from build123d import *

# Parameters (mm, degrees)
F1_DEPTH  = 714.375
F3_D      = 22.225
F3_DEPTH  = 76.2
F3_TIP    = 6.6770636289
F5_DEPTH  = 1792.224
F6_W      = 304.8
F6_H      = 307.975
F7_DEPTH  = 19.05
F10_D     = 22.225
F10_DEPTH = 76.2
F10_TIP   = 6.6770636289
F11_W     = 19.05
F11_H     = 277.495
F12_DEPTH = 304.8
F13_W     = 19.05
F13_H     = 277.495
F14_DEPTH = 304.8
F16_D     = 41.402
F18_DEPTH = 168.402
F19_W     = 304.8
F19_H     = 307.848
F20_DEPTH = 19.05
F22_D     = 28.448
F22_2_D   = 28.448
F24_W     = 19.05
F24_H     = 457.2
F25_DEPTH = 168.402
F27_DEPTH = 1260.349


# Not quite as in the source:
# - a length typed as a fraction of an inch, garbled in the dataset ("3 / 203.2 mm" for 3/8 in), is restored


with BuildPart() as f1:
    # F0 (on Right) → F1 (new body, symmetric)
    with BuildSketch(Plane.YZ):
        with BuildLine():
            Line((152.4, 153.9875), (-152.4, 153.9875))
            Line((-152.4, 153.9875), (-152.4, 138.7475))
            Line((-152.4, 138.7475), (-19.05, 138.7475))
            ThreePointArc((-19.05, 138.7475), (-10.0697438789, 135.0277561211), (-6.35, 126.0475))
            Line((-6.35, 126.0475), (-6.35, -126.0475))
            ThreePointArc((-6.35, -126.0475), (-10.0697438789, -135.0277561211), (-19.05, -138.7475))
            Line((-19.05, -138.7475), (-152.4, -138.7475))
            Line((-152.4, -138.7475), (-152.4, -153.9875))
            Line((-152.4, -153.9875), (152.4, -153.9875))
            Line((152.4, -153.9875), (152.4, -138.7475))
            Line((152.4, -138.7475), (19.05, -138.7475))
            ThreePointArc((19.05, -138.7475), (10.0697438789, -135.0277561211), (6.35, -126.0475))
            Line((6.35, -126.0475), (6.35, 126.0475))
            ThreePointArc((6.35, 126.0475), (10.0697438789, 135.0277561211), (19.05, 138.7475))
            Line((19.05, 138.7475), (152.4, 138.7475))
            Line((152.4, 138.7475), (152.4, 153.9875))
        make_face()
    extrude(amount=F1_DEPTH, both=True)

    # F3
    with Locations(Plane.XY.offset(153.9875)):
        with Locations((-381, 82.55), (-381, -82.55), (171.45, 82.55), (171.45, -82.55), (615.95, 82.55), (615.95, -82.55)):
            Hole(F3_D / 2, depth=F3_DEPTH)
            with Locations((0, 0, -(F3_DEPTH + F3_TIP / 2))):  # 118° drill point
                Cone(0, F3_D / 2, F3_TIP, mode=Mode.SUBTRACT)


with BuildPart() as f5:
    # F4 (on Front) → F5 (new body)
    with BuildSketch(Plane.XZ):
        with BuildLine():
            Line((-47.625, 153.9875), (-352.425, 153.9875))
            Line((-352.425, 153.9875), (-352.425, 138.7475))
            Line((-352.425, 138.7475), (-219.075, 138.7475))
            ThreePointArc((-219.075, 138.7475), (-210.0947438789, 135.0277561211), (-206.375, 126.0475))
            Line((-206.375, 126.0475), (-206.375, -126.0475))
            ThreePointArc((-206.375, -126.0475), (-210.0947438789, -135.0277561211), (-219.075, -138.7475))
            Line((-219.075, -138.7475), (-352.425, -138.7475))
            Line((-352.425, -138.7475), (-352.425, -153.9875))
            Line((-352.425, -153.9875), (-47.625, -153.9875))
            Line((-47.625, -153.9875), (-47.625, -138.7475))
            Line((-47.625, -138.7475), (-180.975, -138.7475))
            ThreePointArc((-180.975, -138.7475), (-189.9552561211, -135.0277561211), (-193.675, -126.0475))
            Line((-193.675, -126.0475), (-193.675, 126.0475))
            ThreePointArc((-193.675, 126.0475), (-189.9552561211, 135.0277561211), (-180.975, 138.7475))
            Line((-180.975, 138.7475), (-47.625, 138.7475))
            Line((-47.625, 138.7475), (-47.625, 153.9875))
        make_face()
    extrude(amount=F5_DEPTH)


with BuildPart() as f5b:
    # F4 (on Front) → F5, piece 2 (new body)
    with BuildSketch(Plane.XZ):
        with BuildLine():
            Line((688.975, 153.9875), (384.175, 153.9875))
            Line((384.175, 153.9875), (384.175, 138.7475))
            Line((384.175, 138.7475), (517.525, 138.7475))
            ThreePointArc((517.525, 138.7475), (526.5052561211, 135.0277561211), (530.225, 126.0475))
            Line((530.225, 126.0475), (530.225, -126.0475))
            ThreePointArc((530.225, -126.0475), (526.5052561211, -135.0277561211), (517.525, -138.7475))
            Line((517.525, -138.7475), (384.175, -138.7475))
            Line((384.175, -138.7475), (384.175, -153.9875))
            Line((384.175, -153.9875), (688.975, -153.9875))
            Line((688.975, -153.9875), (688.975, -138.7475))
            Line((688.975, -138.7475), (555.625, -138.7475))
            ThreePointArc((555.625, -138.7475), (546.6447438789, -135.0277561211), (542.925, -126.0475))
            Line((542.925, -126.0475), (542.925, 126.0475))
            ThreePointArc((542.925, 126.0475), (546.6447438789, 135.0277561211), (555.625, 138.7475))
            Line((555.625, 138.7475), (688.975, 138.7475))
            Line((688.975, 138.7475), (688.975, 153.9875))
        make_face()
    extrude(amount=F5_DEPTH)


with BuildPart() as f7:
    # F6 (on face) → F7 (new body)
    with BuildSketch(Plane.XZ.offset(1792.224)):
        with Locations((-200.025, 0)):
            Rectangle(F6_W, F6_H)
    extrude(amount=F7_DEPTH)


with BuildPart() as f7b:
    # F6 (on face) → F7, piece 2 (new body)
    with BuildSketch(Plane.XZ.offset(1792.224)):
        with Locations((536.575, 0)):
            Rectangle(F6_W, F6_H)
    extrude(amount=F7_DEPTH)


with BuildPart() as f1_1:
    add(f1.part)

    # F8: union F5, F5b, F7b, F7
    add(f5.part)
    add(f5b.part)
    add(f7b.part)
    add(f7.part)

    # F10
    with Locations(Plane.XY.offset(153.9875)):
        with Locations((615.95, -82.55)):
            Hole(F10_D / 2, depth=F10_DEPTH)
            with Locations((0, 0, -(F10_DEPTH + F10_TIP / 2))):  # 118° drill point
                Cone(0, F10_D / 2, F10_TIP, mode=Mode.SUBTRACT)

    # F11 (on face) → F12 (join)
    with BuildSketch(Plane.YZ.offset(688.975)):
        with Locations((-1636.649, 0)):
            Rectangle(F11_W, F11_H)
    extrude(amount=-F12_DEPTH)

    # F13 (on face) → F14 (join)
    with BuildSketch(Plane(origin=(-352.425, 0, 0), x_dir=(0, -1, 0), z_dir=(-1, 0, 0))):
        with Locations((1636.649, 0)):
            Rectangle(F13_W, F13_H)
    extrude(amount=-F14_DEPTH)

    # F16 (through all)
    with Locations(Plane.XY.offset(153.9875)):
        with Locations((619.125, -1739.9), (454.025, -1739.9), (-117.475, -1739.9), (-282.575, -1739.9)):
            Hole(F16_D / 2)


with BuildPart() as f18:
    # F17 (on face) → F18 (new body)
    with BuildSketch(Plane(origin=(0, 0, -153.9875), x_dir=(1, 0, 0), z_dir=(0, 0, -1))):
        with BuildLine():
            Line((-352.425, 420.116), (-352.425, 404.876))
            Line((-352.425, 404.876), (-47.625, 404.876))
            Line((-47.625, 404.876), (-47.625, 420.116))
            Line((-47.625, 420.116), (-180.975, 420.116))
            ThreePointArc((-180.975, 420.116), (-189.9552561211, 423.8357438789), (-193.675, 432.816))
            Line((-193.675, 432.816), (-193.675, 684.784))
            ThreePointArc((-193.675, 684.784), (-189.9552561211, 693.7642561211), (-180.975, 697.484))
            Line((-180.975, 697.484), (-47.625, 697.484))
            Line((-47.625, 697.484), (-47.625, 712.724))
            Line((-47.625, 712.724), (-352.425, 712.724))
            Line((-352.425, 712.724), (-352.425, 697.484))
            Line((-352.425, 697.484), (-219.075, 697.484))
            ThreePointArc((-219.075, 697.484), (-210.0947438789, 693.7642561211), (-206.375, 684.784))
            Line((-206.375, 684.784), (-206.375, 432.816))
            ThreePointArc((-206.375, 432.816), (-210.0947438789, 423.8357438789), (-219.075, 420.116))
            Line((-219.075, 420.116), (-352.425, 420.116))
        make_face()
    extrude(amount=F18_DEPTH)


with BuildPart() as f18b:
    # F17 (on face) → F18, piece 2 (new body)
    with BuildSketch(Plane(origin=(0, 0, -153.9875), x_dir=(1, 0, 0), z_dir=(0, 0, -1))):
        with BuildLine():
            Line((688.975, 420.116), (555.625, 420.116))
            ThreePointArc((555.625, 420.116), (546.6447438789, 423.8357438789), (542.925, 432.816))
            Line((542.925, 432.816), (542.925, 684.784))
            ThreePointArc((542.925, 684.784), (546.6447438789, 693.7642561211), (555.625, 697.484))
            Line((555.625, 697.484), (688.975, 697.484))
            Line((688.975, 697.484), (688.975, 712.724))
            Line((688.975, 712.724), (384.175, 712.724))
            Line((384.175, 712.724), (384.175, 697.484))
            Line((384.175, 697.484), (517.525, 697.484))
            ThreePointArc((517.525, 697.484), (526.5052561211, 693.7642561211), (530.225, 684.784))
            Line((530.225, 684.784), (530.225, 432.816))
            ThreePointArc((530.225, 432.816), (526.5052561211, 423.8357438789), (517.525, 420.116))
            Line((517.525, 420.116), (384.175, 420.116))
            Line((384.175, 420.116), (384.175, 404.876))
            Line((384.175, 404.876), (688.975, 404.876))
            Line((688.975, 404.876), (688.975, 420.116))
        make_face()
    extrude(amount=F18_DEPTH)


with BuildPart() as f20:
    # F19 (on face) → F20 (new body)
    with BuildSketch(Plane(origin=(0, 0, -322.3895), x_dir=(1, 0, 0), z_dir=(0, 0, -1))):
        with Locations((-200.025, 558.8)):
            Rectangle(F19_W, F19_H)
    extrude(amount=F20_DEPTH)

    # F22 (through all)
    with Locations(Plane(origin=(0, 0, -341.4395), x_dir=(1, 0, 0), z_dir=(0, 0, -1))):
        with Locations((-269.1834158416, 628.65), (-130.8665841584, 628.65), (-269.1834158416, 488.95), (-130.8665841584, 488.95), (467.4165841584, 628.65), (605.7334158416, 628.65), (605.7334158416, 488.95), (467.4165841584, 488.95)):
            Hole(F22_D / 2)


with BuildPart() as f20b:
    # F19 (on face) → F20, piece 2 (new body)
    with BuildSketch(Plane(origin=(0, 0, -322.3895), x_dir=(1, 0, 0), z_dir=(0, 0, -1))):
        with Locations((536.575, 558.8)):
            Rectangle(F19_W, F19_H)
    extrude(amount=F20_DEPTH)

    # F22#2 (through all)
    with Locations(Plane(origin=(0, 0, -341.4395), x_dir=(1, 0, 0), z_dir=(0, 0, -1))):
        with Locations((-269.1834158416, 628.65), (-130.8665841584, 628.65), (-269.1834158416, 488.95), (-130.8665841584, 488.95), (467.4165841584, 628.65), (605.7334158416, 628.65), (605.7334158416, 488.95), (467.4165841584, 488.95)):
            Hole(F22_2_D / 2)


with BuildPart() as f1_2:
    add(f1_1.part)

    # F23: union F18, F20, F18b, F20b
    add(f18.part)
    add(f20.part)
    add(f18b.part)
    add(f20b.part)

    # F24 (on face) → F25 (join)
    with BuildSketch(Plane(origin=(0, 0, -153.9875), x_dir=(1, 0, 0), z_dir=(0, 0, -1))):
        with Locations((-200.152, 176.276)):
            Rectangle(F24_W, F24_H)
        with Locations((536.448, 176.276)):
            Rectangle(F24_W, F24_H)
    extrude(amount=F25_DEPTH)

    # F26 (on face) → F27 (cut, through all)
    with BuildSketch(Plane.YZ.offset(545.973)):
        Polygon((52.324, -322.3895), (52.324, -217.4875), (-404.876, -322.3895), align=None)
    extrude(amount=-F27_DEPTH, mode=Mode.SUBTRACT)


solid = f1_2.part
Can you work these out from the model? Positions are in its coordinate system, mm. A direction names the side the tool comes from. Round coordinates to 2 decimals unless told otherwise and drop trailing zeros. Use one line per item in the form item = value. Start each with the question number.
Q1. Which directions (+Z, -Z, +X, -X, +Y, -Y) give clear straight access to the entire face, cutting with the end or side of a thin tool? Please do faces 1 (the face through (-280, -1792.224, 2)), 2 (the face through (-236, -404.876, -246)), 3 (the face through (-202, -1254, -153.988)), 4 (the face through (623, -420.116, -237)), 5 (the face through (450, -1718, 138.748)).
Q2. If I drill on probe 1 along Z at (x, y) = (-251, -583.5); probe 2 along Y at (x, z) = (-51.5, 111); probe 3 along X at (y, z) = (-1739.9, -150.5) (3 decimals), over which ranges is the centre line in solid material (lowest first)? Write a range as [from, to].
Q3. We'd pull the mould along X, two halves only. Please class faces 6 (the face through (-206.375, -805, 2)), 7 (the face through (-279.88, -1719.375, -146.474)), 8 (the face through (618, -812, -138.748)): +X half, -X half, draft (parallel to the pull), parting line (faces both ways), or undercut.
Q4. I'm going to push flat-ended pins straight in: P1, Ø4, axis at y = -1045.5, z = -43.5, coming from the +X side (3 decimals); P2, Ø6, axis at x = 209.5, z = -102, coming from the -Y side; P3, Ø10, axis at x = 413, z = -13, coming from the +Y side. Where does each tip first touch, or does it pass through?
Q5. Imagine slicing it at B-B (y = -1739.9). Count the separate pieces of the cut face and the enclosed holes in it, then the cut area to 3 significant figures.
Worked out:
q1.face_1 = -X
q1.face_2 = -Z, +Y
q1.face_3 = -Z, +X, -X, -Y
q1.face_4 = +X
q1.face_5 = none
q2.probe_1 = [-341.44, -322.39], [-153.99, -138.75], [138.75, 153.99]
q2.probe_2 = [-1811.27, -1792.22], [-1646.17, -1627.12], [-6.35, 6.35]
q2.probe_3 = [-352.425, -303.276], [-261.874, -138.176], [-96.774, -47.625], [384.175, 433.324], [474.726, 598.424], [639.826, 688.975]
q3.face_6 = -X half
q3.face_7 = undercut
q3.face_8 = draft
q4.P1 = 542.925
q4.P2 = -6.35
q4.P3 = 6.35
q5.separate_pieces = 10
q5.enclosed_holes = 0
q5.area = 20,900 mm^2
